Could you check a few things on this model? Use its own coordinates, in mm. Face numbers are marked on the shaded views. A direction names the side the tool comes from. Give positions to 0.01 mm unless a question says otherwise; leave off trailing zeros. Answer in a Markdown table with one row per item. Add a question column.
1. I'm going to push flat-ended pins straight in: pin 1 Ø3 at (x, y) = (157, -2) entering from -Z; pin 2 Ø1.8 at (x, y) = (-155, -1) entering from +Z; pin 3 Ø2.5 at (y, z) = (6.5, -118) entering from +X. Where does each tip first touch, or does it pass through?
2. Which directions (+Z, -Z, +X, -X, +Y, -Y) give clear straight access to the entire face, cutting with the end or side of a thin tool? Please do the marked faces 1, 2, 3, 4 and 5.
3. I need wall thicknesses on line 1 along Y through (x, z) = (-24, -118); line 2 along Z through (x, y) = (124, 6.5); line 3 along Y through (x, z) = (33, 70). Which ranges of each line are inside material? Lowest first, please. Write a range as from..to.
4. Thinking about a two-plate mould opening in X: for the marked faces 6, 7 and 8, which applies, released by +X, released by -X, zero draft, split by the parting line, or undercut?
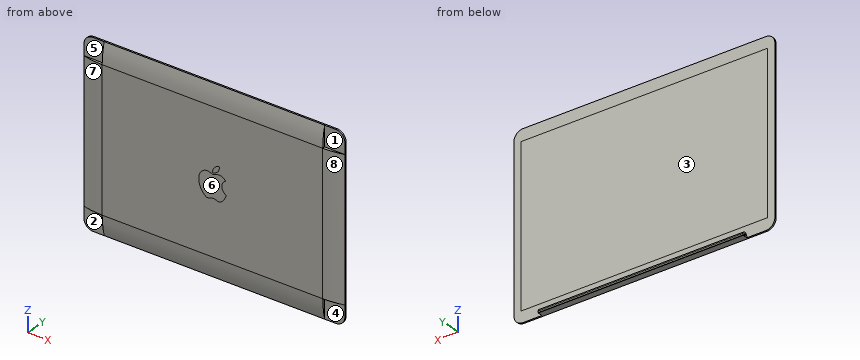
```python
from build123d import *

# Parameters (mm, degrees)
BOSS_EXTRUDE1_DEPTH   = 174.65
BOSS_EXTRUDE2_DEPTH   = 295.3
BOSS_EXTRUDE2_2_DEPTH = 295.3
CUT_EXTRUDE1_DEPTH    = 564.747214252
FILLET1_R             = 12
CUT_EXTRUDE2_DEPTH    = 3.5
SKETCH6_R             = 1
BOSS_EXTRUDE3_DEPTH   = 137.15
SKETCH7_W             = 329.889597284
SKETCH7_H             = 210.188009182
CUT_EXTRUDE3_DEPTH    = 0.0001
CUT_EXTRUDE4_START    = -0.01
CUT_EXTRUDE4_DEPTH    = 0.01


# Read off the part's stored shape, not the designer's step: Cut-Extrude4
with BuildPart() as part:
    # Sketch1 → Boss-Extrude1 (new, symmetric)
    with BuildSketch(Plane(origin=(0, 0, 0), x_dir=(0, 0, -1), z_dir=(1, 0, 0))):
        with BuildLine():
            Line((120.35, 2.092995949), (-120.35, 2.092995949))
            Line((-120.35, 2.092995949), (-120.35, -0.007004051))
            ThreePointArc((-120.35, -0.007004051), (-106.953525194, -2.555626976), (-93.35, -3.507004051))
            Line((-93.35, -3.507004051), (93.35, -3.507004051))
            ThreePointArc((93.35, -3.507004051), (106.953525194, -2.555626976), (120.35, -0.007004051))
            Line((120.35, -0.007004051), (120.35, 2.092995949))
        make_face()
    extrude(amount=BOSS_EXTRUDE1_DEPTH, both=True)


with BuildPart() as body_2:
    # Sketch3 → Boss-Extrude2 (new body)
    with BuildSketch(Plane(origin=(0, 0, -120.35), x_dir=(-1, 0, 0), z_dir=(0, 0, -1))):
        with BuildLine():
            Line((174.65, -3.507004051), (174.65, -0.007004051))
            ThreePointArc((174.65, -0.007004051), (161.253525194, -2.555626976), (147.65, -3.507004051))
            Line((147.65, -3.507004051), (174.65, -3.507004051))
        make_face()
    extrude(amount=BOSS_EXTRUDE2_DEPTH)


with BuildPart() as body_3:
    # Sketch3 → Boss-Extrude2 2 (new body)
    with BuildSketch(Plane(origin=(0, 0, -120.35), x_dir=(-1, 0, 0), z_dir=(0, 0, -1))):
        with BuildLine():
            Line((-174.65, -3.507004051), (-147.65, -3.507004051))
            ThreePointArc((-147.65, -3.507004051), (-161.253525194, -2.555626976), (-174.65, -0.007004051))
            Line((-174.65, -0.007004051), (-174.65, -3.507004051))
        make_face()
    extrude(amount=BOSS_EXTRUDE2_2_DEPTH)


with BuildPart() as cut_extrude1_tool:
    # Sketch4 → Cut-Extrude1 (new, through all)
    with BuildSketch(Plane(origin=(0, 0, -415.65), x_dir=(-1, 0, 0), z_dir=(0, 0, -1))):
        with BuildLine():
            Line((-174.65, -0.007004051), (-174.65, -3.507004051))
            Line((-174.65, -3.507004051), (-147.65, -3.507004051))
            ThreePointArc((-147.65, -3.507004051), (-161.253525194, -2.555626976), (-174.65, -0.007004051))
        make_face()
        with BuildLine():
            Line((174.65, -3.507004051), (174.65, -0.007004051))
            ThreePointArc((174.65, -0.007004051), (161.253525194, -2.555626976), (147.65, -3.507004051))
            Line((147.65, -3.507004051), (174.65, -3.507004051))
        make_face()
    extrude(amount=-CUT_EXTRUDE1_DEPTH)


with BuildPart() as part_1:
    add(part.part)

    # Cut-Extrude1: cut by cut_extrude1_tool
    add(cut_extrude1_tool.part, mode=Mode.SUBTRACT)

    # Fillet1
    fillet1_edges = [part_1.edges().sort_by_distance(p)[0] for p in [
        (-174.65, 1.042995949, 120.35),
        (-174.65, 1.042995949, -120.35),
        (174.65, 1.042995949, -120.35),
        (174.65, 1.042995949, 120.35),
    ]]
    fillet(fillet1_edges, radius=FILLET1_R)

    # Sketch5 → Cut-Extrude2 (cut)
    with BuildSketch(Plane.XZ.offset(3.507004051)):
        Polygon((147.65, -93.35), (210.030677808, -93.35), (147.65, -135.593204027), align=None)
        Polygon((147.65, 93.35), (239.751162266, 93.35), (147.65, 176.927939597), align=None)
        Polygon((-147.65, -93.35), (-147.65, -130.932477463), (-221.764343706, -93.35), align=None)
        Polygon((-147.65, 93.35), (-147.65, 153.997058362), (-221.764343706, 93.35), align=None)
    extrude(amount=-CUT_EXTRUDE2_DEPTH, mode=Mode.SUBTRACT)

    # Sketch6 → Boss-Extrude3 (add, symmetric)
    with BuildSketch(Plane(origin=(0, 0, 0), x_dir=(0, 0, -1), z_dir=(1, 0, 0))):
        with BuildLine():
            Line((118.05, 2.092995949), (118.05, 2.792995949))
            ThreePointArc((118.05, 2.792995949), (115.05, 5.792995949), (118.05, 8.792995949))
            Line((118.05, 8.792995949), (119.85, 8.792995949))
            Line((119.85, 8.792995949), (120.35, 8.692497192))
            Line((120.35, 8.692497192), (120.35, 2.092995949))
            Line((120.35, 2.092995949), (118.05, 2.092995949))
        make_face()
        with Locations((118.05, 5.792995949)):
            Circle(SKETCH6_R, mode=Mode.SUBTRACT)
    extrude(amount=BOSS_EXTRUDE3_DEPTH, both=True)

    # Sketch7 → Cut-Extrude3 (cut)
    with BuildSketch(Plane(origin=(0, 2.092995949, 0), x_dir=(1, 0, 0), z_dir=(0, 1, 0))):
        Rectangle(SKETCH7_W, SKETCH7_H)
    extrude(amount=-CUT_EXTRUDE3_DEPTH, mode=Mode.SUBTRACT)

    # Cut-Extrude4 outline → Cut-Extrude4 (cut)
    with BuildSketch(Plane.XZ.offset(3.507004051).offset(CUT_EXTRUDE4_START)):
        with BuildLine():
            ThreePointArc((-9.086829944, -21.248513597), (-8.191165567, -21.790889583), (-7.183580977, -22.075774961))
            ThreePointArc((-7.183580977, -22.075774961), (-4.970587657, -21.901814224), (-2.834351243, -21.298410749))
            ThreePointArc((-2.834351243, -21.298410749), (1.47428793, -20.400086874), (5.741103254, -21.479736959))
            ThreePointArc((5.741103254, -21.479736959), (9.465377292, -21.935634067), (12.714193917, -20.058601881))
            ThreePointArc((12.714193917, -20.058601881), (14.894750295, -17.768517515), (16.507432012, -15.048486227))
            ThreePointArc((16.507432012, -15.048486227), (17.713556536, -12.779271655), (18.609414677, -10.370639402))
            ThreePointArc((18.609414677, -10.370639402), (12.55251676, -2.119122901), (17.521225226, 6.829925827))
            ThreePointArc((17.521225226, 6.829925827), (13.797071641, 10.184140705), (8.911774187, 11.303938081))
            ThreePointArc((8.911774187, 11.303938081), (6.564348471, 11.150629708), (4.297695677, 10.521188635))
            ThreePointArc((4.297695677, 10.521188635), (2.765098172, 9.975602694), (1.214652309, 9.48302097))
            ThreePointArc((1.214652309, 9.48302097), (0.470107822, 9.356963669), (-0.274436665, 9.48302097))
            ThreePointArc((-0.274436665, 9.48302097), (-2.679371626, 10.302682573), (-5.125261124, 10.990564736))
            ThreePointArc((-5.125261124, 10.990564736), (-7.799066446, 11.233685421), (-10.418034599, 10.642628414))
            ThreePointArc((-10.418034599, 10.642628414), (-14.82861028, 7.663775104), (-17.589225206, 3.113417964))
            ThreePointArc((-17.589225206, 3.113417964), (-18.344964165, -3.082267775), (-17.251311031, -9.22731342))
            ThreePointArc((-17.251311031, -9.22731342), (-14.092597967, -15.865148937), (-9.086829944, -21.248513597))
        make_face()
        with BuildLine():
            ThreePointArc((9.379881835, 21.777318235), (2.623777692, 18.44062415), (0.205889652, 11.303938081))
            ThreePointArc((0.205889652, 11.303938081), (6.961993795, 14.640632167), (9.379881835, 21.777318235))
        make_face()
    extrude(amount=CUT_EXTRUDE4_DEPTH, mode=Mode.SUBTRACT)


with BuildPart() as body_2_1:
    add(body_2.part)

    # Cut-Extrude1: cut by cut_extrude1_tool
    add(cut_extrude1_tool.part, mode=Mode.SUBTRACT)


with BuildPart() as body_3_1:
    add(body_3.part)

    # Cut-Extrude1: cut by cut_extrude1_tool
    add(cut_extrude1_tool.part, mode=Mode.SUBTRACT)


solid = part_1.part
```
Results:
| question | item | result |
|---|---|---|
| 1 | pin 1 | z = -93.35 |
| 1 | pin 2 | z = 93.35 |
| 1 | pin 3 | x = 137.15 |
| 2 | face 1 | +Z, +X, -Y |
| 2 | face 2 | -Z, -X, -Y |
| 2 | face 3 | +Z, +X, -X, +Y |
| 2 | face 4 | -Z, +X, -Y |
| 2 | face 5 | +Z, -X, -Y |
| 3 | line 1 | -0.57..2.09, 2.79..4.79, 6.79..8.79 |
| 3 | line 2 | -120.35..-118.76, -117.34..-115.13 |
| 3 | line 3 | -3.51..2.09 |
| 4 | face 6 | zero draft |
| 4 | face 7 | released by -X |
| 4 | face 8 | released by +X |
